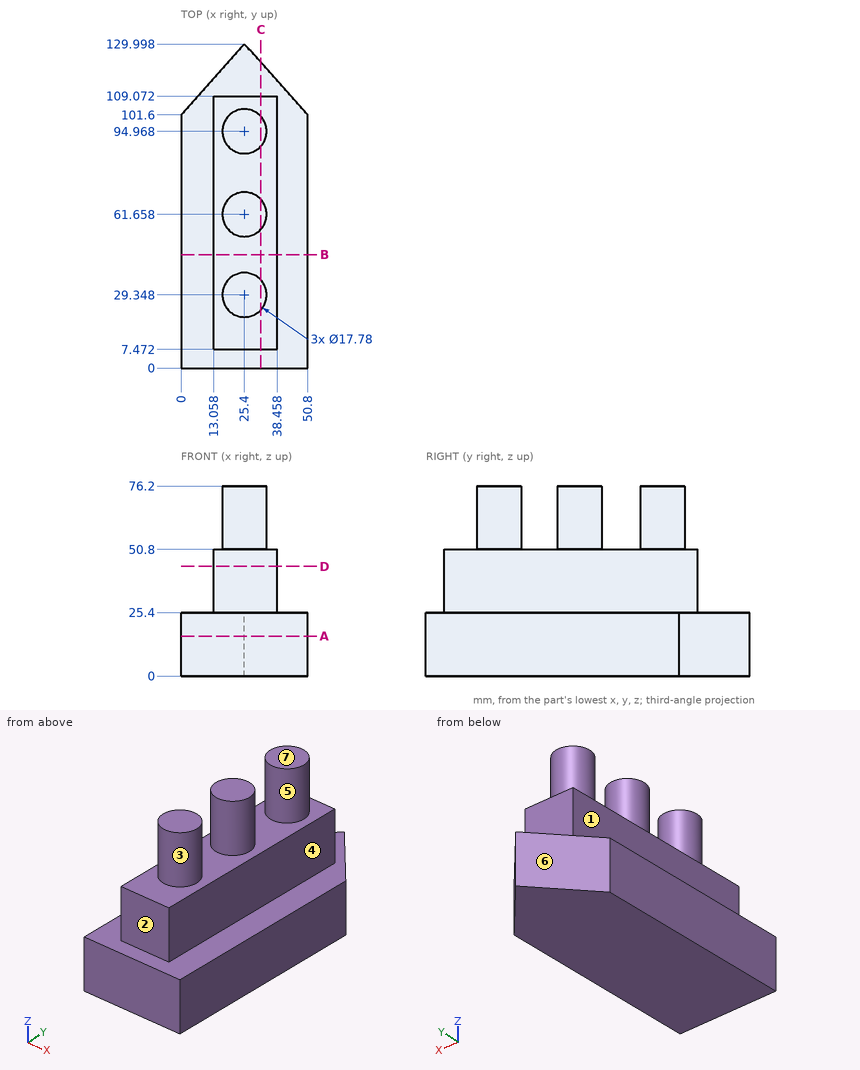
Part print with two shaded views. Sizes in mm from the minimum x, y, z corner. A direction names the side the tool comes from. Round coordinates to 2 decimals unless told otherwise and drop trailing zeros. Order: outer loops, then holes, each group sorted by start corner. A loop starts at its lowest first (then second) coordinate and runs counter-clockwise, first axis right, second up.
(1) 3-axis set-ups, long thin cutter, end or side, ignore diameter. For the marked faces 1, 2, 3 and 4: which of +Z, -Z, +X, -X, +Y, -Y reach the whole face in a straight line?
(2) Band-saw the part on B-B (y = 45.5). List the corners of the cut face in (x, z).
(3) Band-saw the part on C-C (x = 32). List the corners of the cut face in (y, z), then the cut area to 3 significant figures.
(4) Pin check, flat tips, straight feed: pin 1 (8 mm diameter, centred on x = 24, z = 47.5, fed in from +Y); pin 2 (4 mm diameter, centred on x = 8, y = 86, fed in from +Z); pin 3 (7.5 mm diameter, centred on x = 30.5, z = 38.5, fed in from -Y). Stop position of each tip, or through.
(5) Pull direction Y, two halves, no side cores. Call the marked faces 5, 6 and 7: released by +Y, released by -Y, zero draft, split by the parting line, or undercut.
(6) Band-saw the part on D-D (z = 44). List the corners of the cut face in (x, y), then the cut area to 3 significant figures.
(7) Drill centre lines: line 1 (Y direction, x = 25.5, z = 53.5); line 2 (X direction, y = 106, z = 29); line 3 (Z direction, x = 12.5, y = 112). Where is each one in solid material? Low to high.
(8) Band-saw the part on A-A (z = 16). List the corners of the cut face in (x, y), then the cut area to 3 significant figures.
Verdict:
1. face 1: +Z, -X, +Y, -Y
1. face 2: +Z, +X, -X, -Y
1. face 3: +Z
1. face 4: +Z, +X, +Y, -Y
2. outline: (0, 0) - (50.8, 0) - (50.8, 25.4) - (38.46, 25.4) - (38.46, 50.8) - (13.06, 50.8) - (13.06, 25.4) - (0, 25.4) - close
3. outline: (0, 0) - (122.62, 0) - (122.62, 25.4) - (109.07, 25.4) - (109.07, 50.8) - (100.92, 50.8) - (100.92, 76.2) - (89.01, 76.2) - (89.01, 50.8) - (67.61, 50.8) - (67.61, 76.2) - (55.7, 76.2) - (55.7, 50.8) - (35.3, 50.8) - (35.3, 76.2) - (23.39, 76.2) - (23.39, 50.8) - (7.47, 50.8) - (7.47, 25.4) - (0, 25.4) - close
3. area: 6,600 mm2
4. pin 1: stops at y = 109.07
4. pin 2: stops at z = 25.4
4. pin 3: stops at y = 7.47
5. face 5: undercut
5. face 6: released by +Y
5. face 7: zero draft
6. outline: (13.06, 7.47) - (38.46, 7.47) - (38.46, 109.07) - (13.06, 109.07) - close
6. area: 2,580 mm2
7. line 1: y = 20.46 to 38.24, 52.77 to 70.55, 86.08 to 103.86
7. line 2: x = 13.06 to 38.46
7. line 3: z = 0 to 25.4
8. outline: (0, 0) - (50.8, 0) - (50.8, 101.6) - (25.4, 130) - (0, 101.6) - close
8. area: 5,880 mm2
